from build123d import *

# Parameters (mm, degrees)
SKETCH1_R           = 15
BOSS_EXTRUDE1_DEPTH = 35
SKETCH2_R           = 23
BOSS_EXTRUDE2_DEPTH = 7
SKETCH3_R           = 16
BOSS_EXTRUDE3_DEPTH = 25
CUT_EXTRUDE1_DEPTH  = 25


with BuildPart() as part:
    # Sketch1 → Boss-Extrude1 (new body)
    with BuildSketch(Plane.XY):
        Circle(SKETCH1_R)
    extrude(amount=BOSS_EXTRUDE1_DEPTH)

    # Sketch2 → Boss-Extrude2 (add)
    with BuildSketch(Plane.XY.offset(35)):
        Circle(SKETCH2_R)
    extrude(amount=BOSS_EXTRUDE2_DEPTH)

    # Sketch3 → Boss-Extrude3 (add)
    with BuildSketch(Plane.XY.offset(42)):
        Circle(SKETCH3_R)
    extrude(amount=BOSS_EXTRUDE3_DEPTH)

    # Sketch4 → Cut-Extrude1 (cut)
    with BuildSketch(Plane(origin=(0, 10, 0), x_dir=(1, 0, 0), z_dir=(0, 1, 0))):
        with BuildLine():
            Line((5, -24), (5, -9))
            ThreePointArc((5, -9), (0, -4), (-5, -9))
            Line((-5, -9), (-5, -24))
            ThreePointArc((-5, -24), (0, -29), (5, -24))
        make_face()
    extrude(amount=CUT_EXTRUDE1_DEPTH, mode=Mode.SUBTRACT)


solid = part.part
For this review, take the finished solid that the model builds, in its own axes (mm). A direction names the side the tool comes from. Round coordinates to 2 decimals unless told otherwise and drop trailing zeros. Loops run counter-clockwise (first coordinate to the right, second up) from the corner with the lowest first, then second, coordinate; pieces in that order, holes last. Notation, with made-up numbers: (34.25, 12.25) - (91.25, 12.25) arc R29 ccw to (91.25, 48.25) - close; hole circle Ø9 at (-30, 69). An arc over 180 degrees is marked (long way). One line per item, written item: value. Start each with the question number.
Item 1: Take a section at C-C (z = 22.5). Give the boundary of the cut face in (x, y).
Item 2: For faces 4 (the cylindrical face through (-3.47, -15.62, 54.32)), 5 (the flat face through (0, 0, 67)), 6 (the flat face through (0, 10, 16)), 7 (the cylindrical face through (-3.252, -14.643, 17.255)), list the 3-axis set-ups (+Z, -Z, +X, -X, +Y, -Y) from which the entire face can be reached by the end or side of a thin tool; tool diameter is ignored.
Item 3: For L1, parallel to Z at x = -12, y = 9.5; L2, parallel to Z at x = 20.5, y = 9; L3, parallel to X at y = 10.5, z = 23, list the stretches that pass through material, from the lowest coordinate up.
Item 4: Clearance check with flat-ended pins moving along their axes: pin 1 Ø2 at (x, y) = (17, -3) entering from +Z; pin 2 Ø2 at (y, z) = (12.5, 14.5) entering from -X; pin 3 Ø1 at (x, z) = (9.5, 59.5) entering from -Y; pin 4 Ø12 at (x, y) = (-13, 14.5) entering from -Z. State where each tip first meets the part, or that it passes through.
Item 5: Take a section at D-D (x = 0). Give the boundary of the cut face in (y, z), plus the area to 3 significant figures.
Item 6: Take a section at B-B (x = 9.5). Give the boundary of the cut face in (y, z).
Item 7: Take a section at A-A (y = 0). Give the boundary of the cut face in (x, z).
Item 8: The part is to be moulded in two halves that separate along Z. For faces 1 (the flat face through (15, -5, 35)), 2 (the flat face through (-16, -5, 42)), 3 (the flat face through (5, 12, 17)), say which applies: +Z half, -Z half, draft (parallel to the pull), parting line (faces both ways), or undercut.
Answer below:
1. outline: (-5, 10) - (-5, 14.14) arc R15 ccw (long way) to (5, 14.14) - (5, 10) - close
2. face 4: +Z
2. face 5: +Z, +X, -X, +Y, -Y
2. face 6: +Y
2. face 7: -Z
3. L1: z = 35 to 67
3. L2: z = 35 to 42
3. L3: x = -10.71 to -5, 5 to 10.71
4. pin 1: stops at z = 42
4. pin 2: stops at x = -9.63
4. pin 3: stops at y = -13.23
4. pin 4: stops at z = 0
5. outline: (-23, 35) - (-15, 35) - (-15, 0) - (15, 0) - (15, 4) - (10, 4) - (10, 29) - (15, 29) - (15, 35) - (23, 35) - (23, 42) - (16, 42) - (16, 67) - (-16, 67) - (-16, 42) - (-23, 42) - close
5. area: 2,050 mm2
6. outline: (-20.95, 35) - (-11.61, 35) - (-11.61, 0) - (11.61, 0) - (11.61, 35) - (20.95, 35) - (20.95, 42) - (12.87, 42) - (12.87, 67) - (-12.87, 67) - (-12.87, 42) - (-20.95, 42) - close
7. outline: (-23, 35) - (-15, 35) - (-15, 0) - (15, 0) - (15, 35) - (23, 35) - (23, 42) - (16, 42) - (16, 67) - (-16, 67) - (-16, 42) - (-23, 42) - close
8. face 1: -Z half
8. face 2: +Z half
8. face 3: undercut
